from build123d import *

# Parameters (mm, degrees)
BOSS_EXTRUDE1_DEPTH = 5
SHELL1_DEPTH        = 3
DRAFT1_ANGLE        = -25
CUT_EXTRUDE4_DEPTH  = 3
SKETCH7_W           = 2
SKETCH7_H           = 2
BOSS_EXTRUDE3_DEPTH = 6.167458
SKETCH9_W           = 2
SKETCH9_H           = 3
CUT_EXTRUDE5_DEPTH  = 1


# Read off the part's stored shape, not the designer's step: Shell1
with BuildPart() as part:
    # Sketch1 → Boss-Extrude1 (new body)
    with BuildSketch(Plane.XY):
        Polygon((-25.983626021, 33.041313611), (-21.875122617, 59.537949952), (-43.516730546, 62.148416278), (-78.528153024, 63.480237824), (-123.086733491, 63.480237824), (-116.479692334, 29.513255832), (-100.259099485, 29.513255832), (-94.872589048, 10.409344773), (-66.079679944, 10.409344773), (-58.05527459, 29.513255832), (-47.335578993, 29.513255832), align=None)
    extrude(amount=BOSS_EXTRUDE1_DEPTH)

    # Shell1 outline → Shell1 (cut)
    with BuildSketch(Plane.XY):
        Polygon((-47.581760232, 32.513255832), (-27.576866011, 35.818734388), (-24.321805769, 56.811329265), (-43.753778982, 59.155263778), (-78.585191842, 60.480237824), (-119.446966155, 60.480237824), (-114.007006811, 32.513255832), (-97.988004481, 32.513255832), (-92.601494043, 13.409344773), (-68.0734658, 13.409344773), (-60.049060446, 32.513255832), align=None)
    extrude(amount=SHELL1_DEPTH, mode=Mode.SUBTRACT)

    # Draft1
    draft1_faces = [part.faces().sort_by_distance(p)[0] for p in [
        (-52.695426792, 29.513255832, 2.5),
        (-36.659602507, 31.277284722, 2.5),
        (-62.067477267, 19.961300303, 2.5),
        (-80.476134496, 10.409344773, 2.5),
        (-97.565844267, 19.961300303, 2.5),
        (-108.36939591, 29.513255832, 2.5),
        (-119.783212913, 46.496746828, 2.5),
        (-32.695926582, 60.843183115, 2.5),
        (-61.022441785, 62.814327051, 2.5),
        (-100.807443258, 63.480237824, 2.5),
    ]]
    draft(draft1_faces, Plane(origin=(0, 0, 0), x_dir=(-1, 0, 0), z_dir=(0, 0, -1)), DRAFT1_ANGLE)

    # Sketch6 → Cut-Extrude4 (cut)
    with BuildSketch(Plane(origin=(0, 0, 0), x_dir=(-1, 0, 0), z_dir=(0, 0, -1))):
        Polygon((24.321805769, 56.811329265), (22.335064622, 56.571683446), (25.499748774, 36.161943725), (27.576866011, 35.818734388), align=None)
    extrude(amount=-CUT_EXTRUDE4_DEPTH, mode=Mode.SUBTRACT)

    # Sketch7 → Boss-Extrude3 (add)
    with BuildSketch(Plane(origin=(0, 0, 3), x_dir=(-1, 0, 0), z_dir=(0, 0, -1))):
        with Locations((26.823354353, 52.098786124)):
            Rectangle(SKETCH7_W, SKETCH7_H)
        with Locations((26.823354353, 41.748786124)):
            Rectangle(SKETCH7_W, SKETCH7_H)
    extrude(amount=BOSS_EXTRUDE3_DEPTH)

    # Sketch9 → Cut-Extrude5 (cut)
    with BuildSketch(Plane(origin=(0, 0, 3), x_dir=(-1, 0, 0), z_dir=(0, 0, -1))):
        with Locations((80.337479922, 14.909344773)):
            Rectangle(SKETCH9_W, SKETCH9_H)
        with Locations((53.815410339, 34.013255832)):
            Rectangle(SKETCH9_W, SKETCH9_H)
        Polygon((116.917921585, 47.47834949), (113.973113599, 48.051154798), (113.591243393, 46.087949474), (116.53605138, 45.515144166), align=None)
    extrude(amount=-CUT_EXTRUDE5_DEPTH, mode=Mode.SUBTRACT)


solid = part.part
Geometry check sheet. Reference: the model listing, model coordinates, mm. A direction names the side the tool comes from. Round coordinates to 2 decimals unless told otherwise and drop trailing zeros. Order: outer loops, then holes, each group sorted by start corner. A loop starts at its lowest first (then second) coordinate and runs counter-clockwise, first axis right, second up. Notation, with made-up numbers: M 35.5,70.5 L 79.5,70.5 A15 ccw 79.5,97.5 Z; hole C -37.5,-6 d10. An arc over 180 degrees is marked long. Answer in a Markdown table with one row per item. Add a question column.
Item 1: Sectioned sample at C-C, the plane y = 28. Enter the section's corners in (x, z), plus the area to 3 significant figures.
Item 2: Depth check by flat-ended pin: pin 1 Ø4.5 at (x, z) = (-82.5, 2) entering from +Y; pin 2 Ø4 at (x, z) = (-36.5, 3.5) entering from +Y; pin 3 Ø0.5 at (x, z) = (-80, 3.5) entering from -Y; pin 4 Ø6 at (x, y) = (-103.5, 27) entering from +Z. Enter the tip coordinate at first touch or a pass-through.
Item 3: Sectioned sample at A-A, the plane z = -1.5. Enter the section's corners in (x, y).
Item 4: Sectioned sample at B-B, the plane x = -31.5. Enter the section's corners in (y, z), plus the area to 3 significant figures.
Item 5: Draft check along Y on faces 4 (the face through (-106, 32.513, 1)), 5 (the face through (-72, 43, 5)), 6 (the face through (-36.624, 32.448, 2.465)), 7 (the face through (-54, 34, 4)). Enter one of: released by +Y, released by -Y, zero draft, split by the parting line, or undercut.
Item 6: Set-up check for faces 1 (the face through (-116.765, 46.693, 1.528)), 2 (the face through (-100.496, 62.331, 2.465)), 3 (the face through (-27, 40.749, 0)): record each of +Z, -Z, +X, -X, +Y, -Y from which the full face is reachable in a straight line by a thin tool's end or side.
Item 7: Material ranges on L1, parallel to Z at x = -87.5, y = 44.5; L2, parallel to X at y = 21, z = 1.25; L3, parallel to X at y = 19.5, z = 1.5, recorded low to high. Write a range as [from, to].
Filled in:
| question | item | result |
|---|---|---|
| 1 | outline | M -99.83,0 L -96.72,0 L -96.72,3 L -61.94,3 L -61.94,0 L -58.69,0 L -61.22,5 L -97.41,5 Z |
| 1 | area | 89.0 mm² |
| 2 | pin 1 | stops at y = 63.48 |
| 2 | pin 2 | stops at y = 60.63 |
| 2 | pin 3 | stops at y = 11.92 |
| 2 | pin 4 | stops at z = 1.04 |
| 3 | outline | M -27.82,40.75 L -25.82,40.75 L -25.82,42.75 L -27.82,42.75 Z; M -27.82,51.1 L -25.82,51.1 L -25.82,53.1 L -27.82,53.1 Z |
| 4 | outline | M 32.13,0 L 35.17,0 L 35.17,3 L 57.68,3 L 57.68,0 L 60.7,0 L 58.35,5 L 34.49,5 Z |
| 4 | area | 63.5 mm² |
| 5 | face 4 | undercut |
| 5 | face 5 | zero draft |
| 5 | face 6 | released by -Y |
| 5 | face 7 | undercut |
| 6 | face 1 | -Z |
| 6 | face 2 | +Z, +X, -X, +Y |
| 6 | face 3 | -Z, +X |
| 7 | L1 | z = [3, 5] |
| 7 | L2 | x = [-97.25, -94.74], [-64.89, -62.26] |
| 7 | L3 | x = [-96.71, -94.32], [-65.52, -63.02] |
